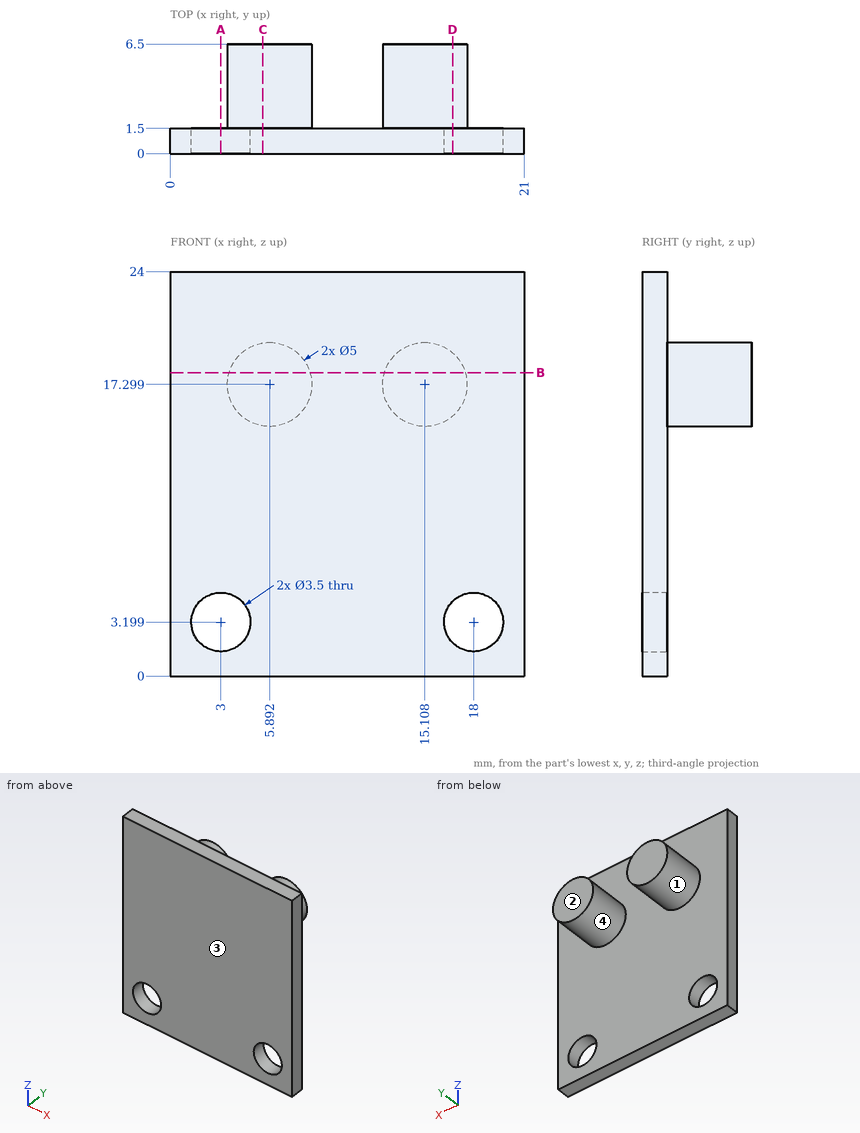
Check sheet for the drawn part. Datum: minimum x, y, z corner. Units: mm. A direction names the side the tool comes from. Round coordinates to 2 decimals unless told otherwise and drop trailing zeros. Order: outer loops, then holes, each group sorted by start corner. A loop starts at its lowest first (then second) coordinate and runs counter-clockwise, first axis right, second up.
1) Scan lines: line 1 (Y direction, x = 9.25, z = 14.75); line 2 (X direction, y = 5.75, z = 15.75) (1 decimal); line 3 (Z direction, x = 17, y = 1) (1 decimal). Record each from-to range of solid material in increasing order.
2) Section check B-B (z = 18). Record the boundary of the cut face in (x, y).
3) Go/stop test with flat-tipped pins: pin 1 Ø3 at (x, y) = (4, 5) entering from -Z; pin 2 Ø2 at (x, z) = (12, 6.5) entering from +Y; pin 3 Ø10 at (x, z) = (17.5, 6) entering from -Y. Record where each tip stops, or that it passes through.
4) Section check C-C (x = 5.5). Record the boundary of the cut face in (y, z).
5) Section check A-A (x = 3). Record the boundary of the cut face in (y, z).
6) Tool access check on the marked faces 3 and 4. Record the directions out of +Z, -Z, +X, -X, +Y, -Y that give a thin tool (end or side, any length) a straight path to the whole face; none if there is none.
7) Mould release check, pull along X, two halves, no side actions. Record for the marked faces 1 and 2: +X half, -X half, draft (parallel to the pull), parting line (faces both ways), or undercut.
8) Section check D-D (x = 16.75). Record the boundary of the cut face in (y, z) (1 decimal).
Result:
1. line 1: y = 0 to 1.5
1. line 2: x = 3.9 to 7.9, 13.1 to 17.1
1. line 3: z = 0 to 1.8, 4.6 to 24
2. outline: (0, 0) - (21, 0) - (21, 1.5) - (17.51, 1.5) - (17.51, 6.5) - (12.71, 6.5) - (12.71, 1.5) - (8.29, 1.5) - (8.29, 6.5) - (3.49, 6.5) - (3.49, 1.5) - (0, 1.5) - close
3. pin 1: stops at z = 14.83
3. pin 2: stops at y = 1.5
3. pin 3: stops at y = 0
4. outline: (0, 0) - (1.5, 0) - (1.5, 14.83) - (6.5, 14.83) - (6.5, 19.77) - (1.5, 19.77) - (1.5, 24) - (0, 24) - close
5. outline: (0, 0) - (1.5, 0) - (1.5, 1.45) - (0, 1.45) - close; (0, 4.95) - (1.5, 4.95) - (1.5, 24) - (0, 24) - close
6. face 3: +Z, -Z, +X, -X, -Y
6. face 4: +Y
7. face 1: undercut
7. face 2: draft
8. outline: (0, 0) - (1.5, 0) - (1.5, 2) - (0, 2) - close; (0, 4.4) - (1.5, 4.4) - (1.5, 15.4) - (6.5, 15.4) - (6.5, 19.2) - (1.5, 19.2) - (1.5, 24) - (0, 24) - close
